Input: part model. Units: mm. Frame: model coordinates. Coordinates: 2 decimals unless noted, no trailing zeros. Loops run counter-clockwise (first coordinate to the right, second up) from the corner with the lowest first, then second, coordinate; pieces in that order, holes last. Notation, with made-up numbers: (27, 50.25) - (57, 50.25) arc R20 ccw to (57, 66.25) - close; hole circle Ø8 at (83.25, 76.25). An arc over 180 degrees is marked (long way). Use a Markdown table: item, result. Add a question column.
1. Contact query for flat-ended pins moving along their axis: P1, Ø1, axis at x = -86, z = 5, coming from the -Y side; P2, Ø10, axis at y = 442, z = 7, coming from the -X side; P3, Ø3, axis at y = 21.5, z = 1.5, coming from the +X side (3 decimals); P4, Ø10, axis at y = 56.5, z = -3.5, coming from the -X side (3 decimals). Output: stop coordinate, or through.
2. Draft query along Z for faces 1 (the face through (-120.464, 242.394, -0.383)), 2 (the face through (-102.675, 242.394, -2.861)), 3 (the face through (4.14, -167.12, 2.78)). Return one class per face: released by +Z, released by -Z, zero draft, split by the parting line, or undercut.
3. Ray query, L1, parallel to Z at x = -111.76, y = 274 (3 decimals); L2, parallel to Z at x = -110.5, y = 419.5; L3, parallel to X at y = 262, z = 1. Return the intervals inside material, ascending. Write a range as [from, to].
4. Section query B-B on y = 391. Return the cut outline in (x, z) (3 decimals), then the cut area to 3 significant figures.
```python
from build123d import *

# Parameters (mm, degrees)
SKETCH2_R   = 9.525
SKETCH2_R_2 = 8.7122


with BuildPart() as part:
    # Sweep1: sweep along a path in Sketch1
    with BuildLine(Plane.XY) as sweep1_path:
        Line((-1.817951031, -173.080098969), (-100.600768363, -74.297281637))
        ThreePointArc((-100.600768363, -74.297281637), (-108.859810189, -61.936752047), (-111.76, -47.356513274))
        Line((-111.76, -47.356513274), (-111.76, 524.143486726))
    # Sketch2 → Sweep1 (sweep)
    with BuildSketch(Plane(origin=(0, 0, 0), x_dir=(1, 0, 0), z_dir=(0, 1, 0))):
        with Locations((-111.76, 0)):
            Circle(SKETCH2_R)
        with Locations((-111.76, 0)):
            Circle(SKETCH2_R_2, mode=Mode.SUBTRACT)
    sweep(path=sweep1_path.line)


solid = part.part
```
Resolved:
| question | item | result |
|---|---|---|
| 1 | P1 | y = -101.01 |
| 1 | P2 | x = -121.07 |
| 1 | P3 | x = -102.235 |
| 1 | P4 | x = -121.285 |
| 2 | face 1 | undercut |
| 2 | face 2 | split by the parting line |
| 2 | face 3 | zero draft |
| 3 | L1 | [-9.525, -8.712], [8.712, 9.525] |
| 3 | L2 | [-9.44, -8.62], [8.62, 9.44] |
| 3 | L3 | [-121.23, -120.41], [-103.11, -102.29] |
| 4 | outline | circle Ø19.05 at (-111.76, 0); hole circle Ø17.424 at (-111.76, 0) |
| 4 | area | 46.6 mm² |
